```python
from build123d import *

# Parameters (mm, degrees)
SKETCH1_W                = 108
SKETCH1_H                = 68
SKETCH1_R                = 2
BOSS_EXTRUDE1_DEPTH      = 3
SKETCH2_W                = 114
SKETCH2_H                = 74
SKETCH2_W_2              = 108
SKETCH2_H_2              = 68
BOSS_EXTRUDE2_DEPTH      = 20
BOSS_EXTRUDE2_DEPTH_BACK = 3
SKETCH4_W                = 111
SKETCH4_H                = 71
SKETCH4_W_2              = 108
SKETCH4_H_2              = 68
BOSS_EXTRUDE3_DEPTH      = 2
CUT_EXTRUDE1_DEPTH       = 4
SKETCH6_R                = 4
SKETCH6_R_2              = 2
BOSS_EXTRUDE4_DEPTH      = 5
SKETCH7_W                = 7
SKETCH7_H                = 7
CUT_EXTRUDE2_DEPTH       = 4
BOSS_EXTRUDE5_DEPTH      = 2


with BuildPart() as part:
    # Sketch1 → Boss-Extrude1 (new body)
    with BuildSketch(Plane(origin=(0, 0, 0), x_dir=(1, 0, 0), z_dir=(0, 1, 0))):
        Rectangle(SKETCH1_W, SKETCH1_H)
        with Locations((-47.1, 27.655555556)):
            Circle(SKETCH1_R, mode=Mode.SUBTRACT)
        with Locations((47.1, 27.655555556)):
            Circle(SKETCH1_R, mode=Mode.SUBTRACT)
        with Locations((47.1, -27.655555556)):
            Circle(SKETCH1_R, mode=Mode.SUBTRACT)
        with Locations((-47.1, -27.655555556)):
            Circle(SKETCH1_R, mode=Mode.SUBTRACT)
    extrude(amount=BOSS_EXTRUDE1_DEPTH)

    # Sketch2 → Boss-Extrude2 (add, two sides)
    with BuildSketch(Plane(origin=(0, 3, 0), x_dir=(1, 0, 0), z_dir=(0, 1, 0))) as boss_extrude2_sk:
        Rectangle(SKETCH2_W, SKETCH2_H)
        Rectangle(SKETCH2_W_2, SKETCH2_H_2, mode=Mode.SUBTRACT)
    extrude(amount=BOSS_EXTRUDE2_DEPTH)
    extrude(boss_extrude2_sk.sketch, amount=-BOSS_EXTRUDE2_DEPTH_BACK)

    # Sketch4 → Boss-Extrude3 (add)
    with BuildSketch(Plane(origin=(0, 23, 0), x_dir=(1, 0, 0), z_dir=(0, 1, 0))):
        Rectangle(SKETCH4_W, SKETCH4_H)
        Rectangle(SKETCH4_W_2, SKETCH4_H_2, mode=Mode.SUBTRACT)
    extrude(amount=BOSS_EXTRUDE3_DEPTH)

    # Sketch5 → Cut-Extrude1 (cut, through all)
    with BuildSketch(Plane.ZY.offset(-54)):
        with BuildLine():
            Line((3, 3), (8, 3))
            Line((8, 3), (8, 6.5))
            ThreePointArc((8, 6.5), (7.560660172, 7.560660172), (6.5, 8))
            Line((6.5, 8), (4.5, 8))
            ThreePointArc((4.5, 8), (3.439339828, 7.560660172), (3, 6.5))
            Line((3, 6.5), (3, 3))
        make_face()
        with BuildLine():
            Line((18, 3), (23, 3))
            Line((23, 3), (23, 6.5))
            ThreePointArc((23, 6.5), (22.560660172, 7.560660172), (21.5, 8))
            Line((21.5, 8), (19.5, 8))
            ThreePointArc((19.5, 8), (18.439339828, 7.560660172), (18, 6.5))
            Line((18, 6.5), (18, 3))
        make_face()
    cut_extrude1 = extrude(amount=-CUT_EXTRUDE1_DEPTH, mode=Mode.SUBTRACT)

    # Sketch6 → Boss-Extrude4 (add)
    with BuildSketch(Plane(origin=(0, 3, 0), x_dir=(1, 0, 0), z_dir=(0, 1, 0))):
        with Locations((-47.1, 27.655555556)):
            Circle(SKETCH6_R)
        with Locations((-47.1, 27.655555556)):
            Circle(SKETCH6_R_2, mode=Mode.SUBTRACT)
        with Locations((47.1, 27.655555556)):
            Circle(SKETCH6_R)
        with Locations((47.1, 27.655555556)):
            Circle(SKETCH6_R_2, mode=Mode.SUBTRACT)
        with Locations((47.1, -27.655555556)):
            Circle(SKETCH6_R)
        with Locations((47.1, -27.655555556)):
            Circle(SKETCH6_R_2, mode=Mode.SUBTRACT)
        with Locations((-47.1, -27.655555556)):
            Circle(SKETCH6_R)
        with Locations((-47.1, -27.655555556)):
            Circle(SKETCH6_R_2, mode=Mode.SUBTRACT)
    extrude(amount=BOSS_EXTRUDE4_DEPTH)

    # Sketch7 → Cut-Extrude2 (cut, through all)
    with BuildSketch(Plane(origin=(0, 3, 0), x_dir=(1, 0, 0), z_dir=(0, 1, 0))):
        with Locations((-10.5, 15.5)):
            Rectangle(SKETCH7_W, SKETCH7_H)
        with Locations((-28.5, 15.5)):
            Rectangle(SKETCH7_W, SKETCH7_H)
        with Locations((7.5, 15.5)):
            Rectangle(SKETCH7_W, SKETCH7_H)
        with Locations((25.5, 15.5)):
            Rectangle(SKETCH7_W, SKETCH7_H)
        with Locations((-10.5, 0.5)):
            Rectangle(SKETCH7_W, SKETCH7_H)
        with Locations((7.5, 0.5)):
            Rectangle(SKETCH7_W, SKETCH7_H)
        with Locations((25.5, 0.5)):
            Rectangle(SKETCH7_W, SKETCH7_H)
        with Locations((-10.5, -14.5)):
            Rectangle(SKETCH7_W, SKETCH7_H)
        with Locations((7.5, -14.5)):
            Rectangle(SKETCH7_W, SKETCH7_H)
        with Locations((25.5, -14.5)):
            Rectangle(SKETCH7_W, SKETCH7_H)
        with Locations((-28.5, 0.5)):
            Rectangle(SKETCH7_W, SKETCH7_H)
        with Locations((-28.5, -14.5)):
            Rectangle(SKETCH7_W, SKETCH7_H)
    extrude(amount=-CUT_EXTRUDE2_DEPTH, mode=Mode.SUBTRACT)

    # Mirror1: Cut-Extrude1 across plane
    add(cut_extrude1.mirror(Plane(origin=(0, 0, 0), x_dir=(0, 0, 1), z_dir=(1, 0, 0))), mode=Mode.SUBTRACT)

    # Sketch8 → Boss-Extrude5 (add)
    with BuildSketch(Plane(origin=(0, 25, 0), x_dir=(1, 0, 0), z_dir=(0, 1, 0))):
        Polygon((55.5, 35.5), (50.5, 35.5), (50.5, 34), (54, 34), (54, 30.5), (55.5, 30.5), align=None)
        Polygon((-55.5, -35.5), (-50.5, -35.5), (-50.5, -34), (-54, -34), (-54, -30.5), (-55.5, -30.5), align=None)
    extrude(amount=BOSS_EXTRUDE5_DEPTH)


solid = part.part
```
Work out the finished part from the listing and answer in its coordinate system (mm). A direction names the side the tool comes from. Coordinates: 2 decimals unless noted, no trailing zeros. Loops run counter-clockwise (first coordinate to the right, second up) from the corner with the lowest first, then second, coordinate; pieces in that order, holes last. Notation, with made-up numbers: M 10.5,6 L 17.5,6 A9 ccw 17.5,17 Z; hole C -38,88.25 d3. An arc over 180 degrees is marked long. Use CSV: the item, a comma, the result in double quotes. Start each with the question number.
(1) For faces 1 (the face through (45, 8, -27)), 2 (the face through (-1, 0, -1)), 3 (the face through (-55, 5, 3)), 4 (the face through (11, 2, -15)), determine the directions among +Z, -Z, +X, -X, +Y, -Y from which every point of the face is accessible in a straight line to the end or side of a thin tool.
(2) Given pin 1 Ø3 at (x, y) = (-5, 25) entering from +Z; pin 2 Ø5 at (x, z) = (-1, -17) entering from +Y; pin 3 Ø4.5 at (y, z) = (25.5, -11.5) entering from -X; pin 4 Ø1.2 at (x, y) = (26, 26) entering from -Z, each flat-ended and moving along its own axis, determine where each tip first touches the part or whether it passes through.
(3) Find section A-A, the plane x = 47.1. Give the vertices of the cut face in (y, z), then the cut area to 3 significant figures.
(4) Find section C-C, the plane x = 27. Give the vertices of the cut face in (y, z), then the cut area to 3 significant figures.
(5) Find section B-B, the plane y = 18. Give the vertices of the cut face in (x, z).
(6) Consider line 1 (Z direction, x = 47.1, y = 3.25); line 2 (X direction, y = 9, z = -12); line 3 (Z direction, x = -23, y = 23.25). Determine where each line is inside the solid, lowest interval first.
(7) Find section D-D, the plane z = -1.5. Give the vertices of the cut face in (x, y), then the cut area to 3 significant figures.
(8) For a pull along X with two mould halves and no side action, classify faces 5 (the face through (-57, 12, 1)), 6 (the face through (1, 24, -35.5)), 7 (the face through (25, 2, -19)) as +X half, -X half, draft (parallel to the pull), parting line (faces both ways), or undercut.
Recorded:
1,face 1,"+Y"
1,face 2,"+Z, -Z, +X, -X, -Y"
1,face 3,"+X, -X"
1,face 4,"+Y, -Y"
2,pin 1,"stops at z = 35.5"
2,pin 2,"stops at y = 3"
2,pin 3,"stops at x = -55.5"
2,pin 4,"passes through"
3,outline,"M 0,-37 L 23,-37 L 23,-35.5 L 25,-35.5 L 25,-34 L 3,-34 L 3,-31.66 L 8,-31.66 L 8,-29.66 L 0,-29.66 Z; M 0,-25.66 L 8,-25.66 L 8,-23.66 L 3,-23.66 L 3,23.66 L 8,23.66 L 8,25.66 L 0,25.66 Z; M 0,29.66 L 8,29.66 L 8,31.66 L 3,31.66 L 3,34 L 25,34 L 25,35.5 L 23,35.5 L 23,37 L 0,37 Z"
3,area,"364 mm^2"
4,outline,"M 0,-37 L 23,-37 L 23,-35.5 L 25,-35.5 L 25,-34 L 3,-34 L 3,-19 L 0,-19 Z; M 0,-12 L 3,-12 L 3,-4 L 0,-4 Z; M 0,3 L 3,3 L 3,11 L 0,11 Z; M 0,18 L 3,18 L 3,34 L 25,34 L 25,35.5 L 23,35.5 L 23,37 L 0,37 Z"
4,area,"285 mm^2"
5,outline,"M -57,-37 L 57,-37 L 57,37 L -57,37 Z; hole M -54,-34 L 54,-34 L 54,34 L -54,34 Z"
6,line 1,"z = -37 to -34, -31.66 to -29.66, -25.66 to -23.66, 23.66 to 25.66, 29.66 to 31.66, 34 to 37"
6,line 2,"x = -57 to -54, 54 to 57"
6,line 3,"z = -35.5 to -34, 34 to 35.5"
7,outline,"M -57,0 L -32,0 L -32,3 L -54,3 L -54,25 L -55.5,25 L -55.5,23 L -57,23 Z; M -25,0 L -14,0 L -14,3 L -25,3 Z; M -7,0 L 4,0 L 4,3 L -7,3 Z; M 11,0 L 22,0 L 22,3 L 11,3 Z; M 29,0 L 57,0 L 57,23 L 55.5,23 L 55.5,25 L 54,25 L 54,3 L 29,3 Z"
7,area,"384 mm^2"
8,face 5,"-X half"
8,face 6,"draft"
8,face 7,"undercut"
